Could you check a few things on this model? Use its own coordinates, in mm. A direction names the side the tool comes from. Give positions to 0.01 mm unless a question says otherwise; leave off trailing zeros. Order: outer loops, then holes, each group sorted by start corner. A loop starts at its lowest first (then second) coordinate and runs counter-clockwise, first axis right, second up. Notation, with made-up numbers: (80.25, -40) - (99.25, -40) arc R33 cw to (99.25, -10) - close; hole circle Ø6 at (43, -38). An arc over 180 degrees is marked (long way). Put each result on its own line as item: value.
Autodesk Inventor part; units mm, degrees
ref_plane "Plano de trabajo2" through (0, -18.5, 0) normal (0, 1, 0) x (1, 0, 0)
ref_plane "YZ Plane" through (0, 0, 0) normal (1, 0, 0) x (0, 1, 0)
ref_plane "XZ Plane" through (0, 0, 0) normal (0, 1, 0) x (-1, 0, 0)
sketch "Boceto1" plane through (0, 0, 0) normal (0, 1, 0) x (-1, 0, 0)
  circle A0 centre (0, 0) radius 9
  circle A1 centre (0, 0) radius 13.325
  dimension "d0" = 18
  dimension "d1" = 26.65
extrude "Extrusión1" add sketch "Boceto1" against normal blind 23.6
ref_plane "Plano de trabajo2" through (0, -18.5, 0) normal (0, 1, 0) x (1, 0, 0)
sketch "Boceto4" plane through (0, -18.5, 0) normal (0, 1, 0) x (1, 0, 0)
  circle A0 centre (0, 0) radius 6.8
  dimension "d18" = 13.6
extrude "Extrusión4" add sketch "Boceto4" against normal blind 18.97
sketch "Boceto5" plane through (0, 0, 0) normal (0, 1, 0) x (1, 0, 0)
  circle A0 centre (0, 0) radius 10.7
extrude "Extrusión5" cut sketch "Boceto5" against normal blind 18.97
sketch "Boceto6" plane through (0, -37.47, 0) normal (0, -1, 0) x (1, 0, 0)
  circle A0 centre (0, 0) radius 6.7
  circle A1 centre (0, 0) radius 9.3
  dimension "d25" = 13.4
  dimension "d26" = 18.6
extrude "Extrusión6" add sketch "Boceto6" against normal blind 18.97
sketch "Boceto7" plane through (0, -37.47, 0) normal (0, -1, 0) x (1, 0, 0)
  circle A0 centre (0, 0) radius 8.5
  dimension "d29" = 17
extrude "Extrusión7" cut sketch "Boceto7" against normal blind 18.97
thread "Rosca2"
sketch "Boceto9" plane through (0, -37.47, 0) normal (0, -1, 0) x (1, 0, 0)
  circle A0 centre (0, 0) radius 9.3
extrude "Extrusión8" cut sketch "Boceto9" along normal blind 8.47
sketch "Boceto10" plane through (0, -23.6, 0) normal (0, -1, 0) x (1, 0, 0)
  circle A0 centre (0, 0) radius 10.7
extrude "Extrusión9" add sketch "Boceto10" against normal blind 1
sketch "Boceto11" plane through (0, -23.6, 0) normal (0, -1, 0) x (1, 0, 0)
  circle A0 centre (0, 0) radius 8.5
extrude "Extrusión10" cut sketch "Boceto11" against normal blind 53.22
sketch "Boceto12" plane through (0, 0, 0) normal (0, 1, 0) x (1, 0, 0)
  circle A0 centre (0, 0) radius 8.5
  circle A1 centre (0, 0) radius 10.7
  circle A2 centre (0, 0) radius 9.3
  circle A3 centre (0, 0) radius 13.88
extrude "Extrusión11" cut sketch "Boceto12" against normal blind 8.47 contours A3
sketch "Boceto13" plane through (0, -8.47, 0) normal (0, 1, 0) x (1, 0, 0)
  circle A0 centre (0, 0) radius 10.7
  circle A1 centre (0, 0) radius 10.7
extrude "Extrusión12" add sketch "Boceto13" against normal up to surface (15.13 mm away)
sketch "Boceto14" plane through (0, -37.47, 0) normal (0, -1, 0) x (1, 0, 0)
  circle A0 centre (0, 0) radius 8.5
  circle A1 centre (0, 0) radius 8.5
extrude "Extrusión13" add sketch "Boceto14" against normal up to surface (13.87 mm away)
sketch "Boceto15" plane through (0, -37.47, 0) normal (0, -1, 0) x (1, 0, 0)
  circle A0 centre (0, 0) radius 9.3
  circle A1 centre (0, 0) radius 9.3
  dimension "d46" = 18.6
properties part number "Acople con rosca" material "PVC, no plastificado"
1) Suppose I cut it at A-A, the plane x = 0. List the corners of the cut face in (y, z) for me (3 decimals), and give its area (3 significant figures).
Filled in:
outline: (-37.47, -9.3) - (-23.6, -9.3) - (-23.6, -13.325) - (-8.47, -13.325) - (-8.47, 13.325) - (-23.6, 13.325) - (-23.6, 9.3) - (-37.47, 9.3) - close
area: 661 mm^2
2) Suppose I cut it at B-B, the plane z = 0. List the corners of the cut face in (x, y) for me (3 decimals).
Filled in:
outline: (-13.325, -23.6) - (-9.3, -23.6) - (-9.3, -37.47) - (9.3, -37.47) - (9.3, -23.6) - (13.325, -23.6) - (13.325, -8.47) - (-13.325, -8.47) - close
3) Which directions (+Z, -Z, +X, -X, +Y, -Y) give clear straight access to the entire face, cutting with the end or side of a thin tool? Please do faces 1 (the flat face through (-3, -23.6, 9)), 2 (the flat face through (0, -37.47, 0)).
Filled in:
face 1: -Y
face 2: +Z, -Z, +X, -X, -Y
4) If I drill on line 1 (Y direction, x = 6, z = -11.5); line 2 (Z direction, x = -9.25, y = -12.25); line 3 (Z direction, x = 0, y = -15.25) (3 decimals), over which ranges is the centre line in solid material (lowest first)? Write a range as [from, to].
Filled in:
line 1: y = [-23.6, -8.47]
line 2: z = [-9.59, 9.59]
line 3: z = [-13.325, 13.325]
5) I'm going to push flat-ended pins straight in: pin 1 (12 mm diameter, centred on x = -7, y = -32, fed in from +Z); pin 2 (10 mm diameter, centred on x = 10.5, y = -31, fed in from +Z); pin 3 (8 mm diameter, centred on x = -7.5, y = -11.5, fed in from +Z). Where does each tip first touch, or does it pass through?
Filled in:
pin 1: stops at z = 9.25
pin 2: stops at z = 7.5
pin 3: stops at z = 12.86
6) Suppose I cut it at D-D, the plane y = -22. List the corners of the cut face in (x, z) for me (3 decimals).
Filled in:
outline: circle Ø26.65 at (0, 0)
7) Suppose I cut it at C-C, the plane y = -26.75. List the corners of the cut face in (x, z) for me, and give its area (3 significant figures).
Filled in:
outline: circle Ø18.6 at (0, 0)
area: 272 mm^2
